Answer from the drawing. Dimensions are ordinates in mm from the lowest x, y and z of the part. Give positions to 0.01 mm unless a question says otherwise; leave off trailing zeros. Loops run counter-clockwise (first coordinate to the right, second up) from the corner with the lowest first, then second, coordinate; pieces in that order, holes last. Notation, with made-up numbers: (85, -13.5) - (141, -13.5) arc R17 ccw to (141, -4.5) - close; hole circle Ø7 at (27, -28). An arc over 180 degrees is marked (long way). Write each question's results on one line, items separated by ' | '. Start each with the question number.
Q1. Given pin 1 (5.5 mm diameter, centred on y = 24.8, z = 18.47, fed in from +X), flat-ended and moving along its own axis, determine where the tip first touches the part or whether it passes through.
Q2. The part is cut by section A-A, the plane z = 5.7. Write down the section's boundary in (x, y).
Q3. The part is cut by section D-D, the plane y = 21.25. Write down the section's boundary in (x, z) (1 decimal).
Q4. The part is cut by section C-C, the plane x = 3.2. Write down the section's boundary in (y, z), plus the area to 3 significant figures.
Q5. Determine the mould class of the marked faces 1, 2, 3 and 4 for opening direction Z: +Z half, -Z half, draft (parallel to the pull), parting line (faces both ways), or undercut.
Q6. Find the intervals of material crossed by line 1 (Z direction, x = 1.05, y = 24.8) (1 decimal); line 2 (Z direction, x = 1.2, y = 24) (1 decimal); line 3 (Y direction, x = 0.55, z = 23) (1 decimal), in increasing order. Write a range as from..to.
Q7. The part is cut by section B-B, the plane y = 24.25. Write down the section's boundary in (x, z), plus the area to 3 significant figures.
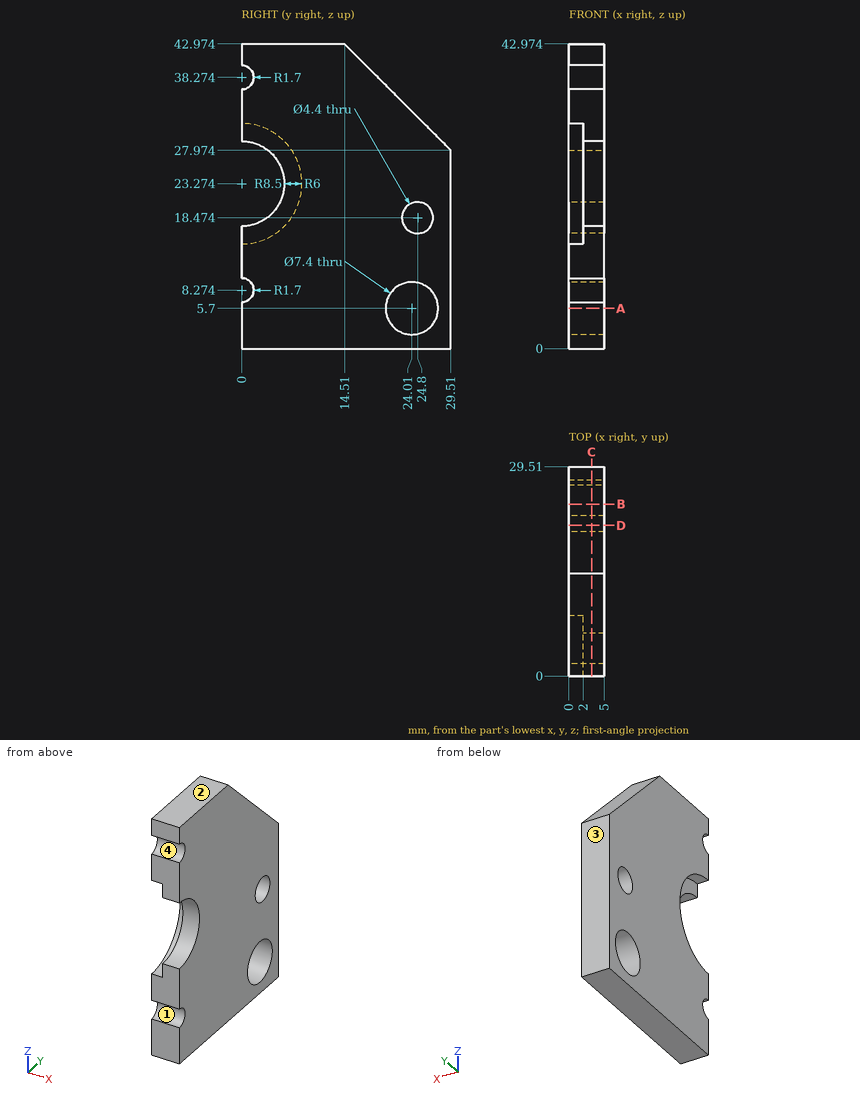
Check sheet entries:
1) pin 1: stops at x = 5
2) outline: (0, 0) - (5, 0) - (5, 20.31) - (0, 20.31) - close; (0, 27.71) - (5, 27.71) - (5, 29.51) - (0, 29.51) - close
3) outline: (0, 0) - (5, 0) - (5, 3.2) - (0, 3.2) - close; (0, 8.2) - (5, 8.2) - (5, 36.2) - (0, 36.2) - close
4) outline: (0, 0) - (29.51, 0) - (29.51, 27.97) - (14.51, 42.97) - (0, 42.97) - (0, 39.97) arc R1.7 cw to (0, 36.57) - (0, 29.27) arc R6 cw to (0, 17.27) - (0, 9.97) arc R1.7 cw to (0, 6.57) - close; hole circle Ø7.4 at (24.01, 5.7); hole circle Ø4.4 at (24.8, 18.47) | area: 1,030 mm^2
5) face 1: undercut | face 2: +Z half | face 3: draft | face 4: undercut
6) line 1: z = 0..2.1, 9.3..16.3, 20.7..32.7 | line 2: z = 0..2, 9.4..16.4, 20.5..33.5 | line 3: y = 8.5..29.5
7) outline: (0, 0) - (5, 0) - (5, 2.01) - (0, 2.01) - close; (0, 9.39) - (5, 9.39) - (5, 16.34) - (0, 16.34) - close; (0, 20.6) - (5, 20.6) - (5, 33.23) - (0, 33.23) - close | area: 108 mm^2
